```python
from build123d import *

# Parameters (mm, degrees)
SKETCH1_R                       = 35
BOSS_EXTRUDE1_DEPTH             = 20
SKETCH2_R                       = 32.5
CUT_EXTRUDE1_DEPTH              = 6.5
SKETCH3_R                       = 31.35
BOSS_EXTRUDE2_DEPTH             = 6.5
BOSS_EXTRUDE3_DEPTH             = 20
SKETCH14_R                      = 14.5
CUT_EXTRUDE2_DEPTH              = 5
SKETCH15_R                      = 13.5
BOSS_EXTRUDE4_DEPTH             = 4
TAP_DRILL_FOR_3_8_16_TAP1_D     = 7.9375
TAP_DRILL_FOR_3_8_16_TAP1_DEPTH = 40
TAP_DRILL_FOR_3_8_16_TAP1_TIP   = 2.384665582
FILLET1_R                       = 1


with BuildPart() as part:
    # Sketch1 → Boss-Extrude1 (new body)
    with BuildSketch(Plane(origin=(0, 0, 0), x_dir=(1, 0, 0), z_dir=(0, 1, 0))):
        with Locations(Location((0, 0, 0), (0, 0, 270))):
            Circle(SKETCH1_R)
    extrude(amount=BOSS_EXTRUDE1_DEPTH)

    # Sketch2 → Cut-Extrude1 (cut)
    with BuildSketch(Plane(origin=(0, 20, 0), x_dir=(1, 0, 0), z_dir=(0, 1, 0))):
        with Locations(Location((0, 0, 0), (0, 0, 270))):
            Circle(SKETCH2_R)
    extrude(amount=-CUT_EXTRUDE1_DEPTH, mode=Mode.SUBTRACT)

    # Sketch3 → Boss-Extrude2 (add)
    with BuildSketch(Plane(origin=(0, 13.5, 0), x_dir=(1, 0, 0), z_dir=(0, 1, 0))):
        with Locations(Location((0, 0, 0), (0, 0, 270))):
            Circle(SKETCH3_R)
    extrude(amount=BOSS_EXTRUDE2_DEPTH)

    # Sketch8 → Boss-Extrude3 (add)
    with BuildSketch(Plane(origin=(0, 0, 0), x_dir=(1, 0, 0), z_dir=(0, 1, 0))):
        with BuildLine():
            ThreePointArc((33.393164213, -10.483157151), (0, -35), (-33.393164213, -10.483157151))
            Line((-33.393164213, -10.483157151), (-10, -85))
            Line((-10, -85), (10, -85))
            Line((10, -85), (33.393164213, -10.483157151))
        make_face()
    extrude(amount=BOSS_EXTRUDE3_DEPTH)

    # Sketch14 → Cut-Extrude2 (cut)
    with BuildSketch(Plane(origin=(0, 20, 0), x_dir=(1, 0, 0), z_dir=(0, 1, 0))):
        with Locations(Location((0, -52, 0), (0, 0, 270))):
            Circle(SKETCH14_R)
    extrude(amount=-CUT_EXTRUDE2_DEPTH, mode=Mode.SUBTRACT)

    # Sketch15 → Boss-Extrude4 (add)
    with BuildSketch(Plane(origin=(0, 15, 0), x_dir=(1, 0, 0), z_dir=(0, 1, 0))):
        with Locations(Location((0, -52, 0), (0, 0, 270))):
            Circle(SKETCH15_R)
    extrude(amount=BOSS_EXTRUDE4_DEPTH)

    # Tap Drill for 3/8-16 Tap1
    with Locations(Plane.XY.offset(85)):
        with Locations((0, 10)):
            Hole(TAP_DRILL_FOR_3_8_16_TAP1_D / 2, depth=TAP_DRILL_FOR_3_8_16_TAP1_DEPTH)
            with Locations((0, 0, -(TAP_DRILL_FOR_3_8_16_TAP1_DEPTH + TAP_DRILL_FOR_3_8_16_TAP1_TIP / 2))):  # 118° drill point
                Cone(0, TAP_DRILL_FOR_3_8_16_TAP1_D / 2, TAP_DRILL_FOR_3_8_16_TAP1_TIP, mode=Mode.SUBTRACT)

    # Fillet1
    fillet1_edges = [part.edges().sort_by_distance(p)[0] for p in [
        (0, 0, -35),
        (-21.696582106, 0, 47.741578576),
        (-10, 10, 85),
        (0, 0, 85),
        (10, 10, 85),
        (21.696582106, 0, 47.741578576),
        (-21.696582106, 20, 47.741578576),
        (0, 20, 85),
        (21.696582106, 20, 47.741578576),
        (0, 20, -35),
    ]]
    fillet(fillet1_edges, radius=FILLET1_R)


solid = part.part
```
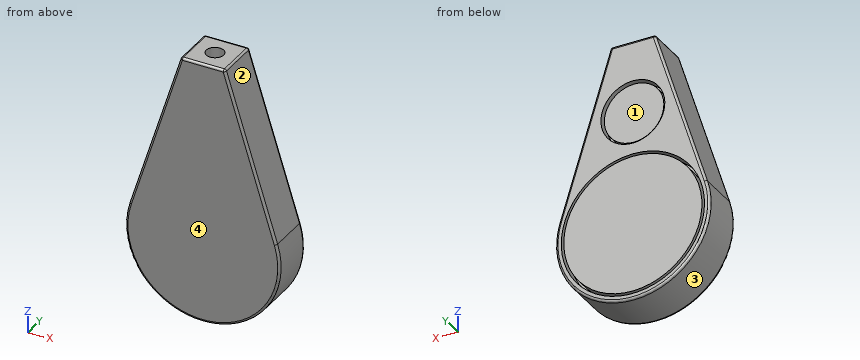
Part model, mm, in its own coordinate system. Face numbers are marked on the shaded views. Round coordinates to 2 decimals unless told otherwise and drop trailing zeros. Answer as CSV lines item,"result". Start each with the question number.
1) Drop flat-ended pins along their axis: pin 1 (5 mm diameter, centred on x = 0, y = 10, fed in from -Z); pin 2 (4 mm diameter, centred on y = 10.5, z = 71, fed in from -X); pin 3 (4 mm diameter, centred on y = 11.5, z = 6, fed in from -X). Give the stop position or say it passes through.
2) Mould opens along Z. For the marked faces 1, 2, 3 and 4 say: +Z half, -Z half, draft (parallel to the pull), parting line (faces both ways), or undercut.
3) Drill centre lines: L1, parallel to X at y = 18.5, z = 0; L2, parallel to X at y = 18.75, z = 52; L3, parallel to X at y = 10, z = 61. Where is each one in solid material? Low to high.
Worked out:
1,pin 1,"z = -35"
1,pin 2,"x = -15.02"
1,pin 3,"x = -34.77"
2,face 1,"undercut"
2,face 2,"+Z half"
2,face 3,"parting line"
2,face 4,"draft"
3,L1,"-35 to -32.5, -31.35 to 31.35, 32.5 to 35"
3,L2,"-20.36 to -14.5, -13.5 to 13.5, 14.5 to 20.36"
3,L3,"-17.53 to -3.97, 3.97 to 17.53"
